Geometry: final body of the model. Coordinates: model frame, mm. A direction names the side the tool comes from. Give positions to 0.01 mm unless a question says otherwise; leave off trailing zeros. Write each loop counter-clockwise with the first axis right and the second up, starting at its lowest first coordinate (ties: lowest second). Pieces come first, ordered by that corner, then holes.
from build123d import *

# Parameters (mm, degrees)
SKETCH1_R           = 1.5
BOSS_EXTRUDE1_DEPTH = 3
SCALE1_SCALE        = 1.8


with BuildPart() as part:
    # Sketch1 → Boss-Extrude1 (new body)
    with BuildSketch(Plane(origin=(0, 0, 0), x_dir=(1, 0, 0), z_dir=(0, 1, 0))):
        with BuildLine():
            Line((0, -5), (23.998875872, -5))
            ThreePointArc((23.998875872, -5), (24.467345461, -4.883479623), (24.826642543, -4.561072489))
            Line((24.826642543, -4.561072489), (28.564941326, 0.954149161))
            ThreePointArc((28.564941326, 0.954149161), (28.766036178, 1.172359953), (29.022312673, 1.321950886))
            Line((29.022312673, 1.321950886), (40.929553216, 6.070049343))
            ThreePointArc((40.929553216, 6.070049343), (41.304486381, 6.141164834), (41.678758689, 6.066649533))
            Line((41.678758689, 6.066649533), (47.144586244, 3.829406729))
            Line((47.144586244, 3.829406729), (48.06174016, 3.086958957))
            Line((48.06174016, 3.086958957), (48.804187932, 4.004112872))
            Line((48.804187932, 4.004112872), (49.721341848, 3.2616651))
            Line((49.721341848, 3.2616651), (50.46378962, 4.178819016))
            Line((50.46378962, 4.178819016), (51.380943536, 3.436371244))
            Line((51.380943536, 3.436371244), (52.123391308, 4.35352516))
            Line((52.123391308, 4.35352516), (53.040545224, 3.611077387))
            Line((53.040545224, 3.611077387), (53.782992996, 4.528231303))
            Line((53.782992996, 4.528231303), (54.700146912, 3.785783531))
            Line((54.700146912, 3.785783531), (55.442594685, 4.702937447))
            Line((55.442594685, 4.702937447), (52.341745918, 12.244834503))
            ThreePointArc((52.341745918, 12.244834503), (52.137055639, 12.558350103), (51.831402108, 12.774604725))
            Line((51.831402108, 12.774604725), (46.024183924, 15.419882568))
            ThreePointArc((46.024183924, 15.419882568), (45.628323444, 15.509674561), (45.229386093, 15.434727162))
            Line((45.229386093, 15.434727162), (20.032711481, 5.075121772))
            ThreePointArc((20.032711481, 5.075121772), (19.846254378, 5.018960187), (19.652448068, 5))
            Line((19.652448068, 5), (0, 5))
            ThreePointArc((0, 5), (-5, 0), (0, -5))
        make_face()
        Circle(SKETCH1_R, mode=Mode.SUBTRACT)
        with Locations((22, 0)):
            Circle(SKETCH1_R, mode=Mode.SUBTRACT)
    extrude(amount=BOSS_EXTRUDE1_DEPTH)


with BuildPart() as part_1:
    # Scale1: scaled about (24.6084342, 1.5, -3.682524739)
    add(part.part.scale(SCALE1_SCALE).moved(Location((-19.68674736, -1.2, 2.946019791))))


solid = part_1.part
Q1. Section B-B on x = 10. Output: boundary loops of the cut face in (y, z), plus the area to 3 significant figures.
Filled sheet:
outline: (-1.2, -6.05) - (4.2, -6.05) - (4.2, 11.95) - (-1.2, 11.95) - close
area: 97.2 mm2
Q2. Section A-A on y = 2.95. Output: boundary loops of the cut face in (x, z).
Filled sheet:
outline: (-19.69, -6.05) - (15.69, -6.05) arc R1.8 cw to (16.37, -6.19) - (61.73, -24.84) arc R1.8 ccw to (63.16, -24.81) - (73.61, -20.05) arc R1.8 ccw to (74.53, -19.09) - (80.11, -5.52) - (78.77, -3.87) - (77.12, -5.2) - (75.79, -3.55) - (74.14, -4.89) - (72.8, -3.24) - (71.15, -4.58) - (69.81, -2.92) - (68.16, -4.26) - (66.82, -2.61) - (65.17, -3.95) - (55.34, -7.97) arc R1.8 cw to (53.99, -7.98) - (32.55, 0.57) arc R1.8 cw to (31.73, 1.23) - (25, 11.16) arc R1.8 ccw to (23.51, 11.95) - (-19.69, 11.95) arc R9 ccw to start; hole circle Ø5.4 at (-19.69, 2.95); hole circle Ø5.4 at (19.91, 2.95)
Q3. Ray query, line 1 along X through (y, z) = (2.6, 2.5); line 2 along Z through (x, y) = (-21.5, 1.8); line 3 along Z through (x, y) = (0.5, 2.35). Return the intervals inside material, ascending.
Filled sheet:
line 1: x = -28.68 to -22.35, -17.02 to 17.25, 22.58 to 30.87
line 2: z = -5.87 to 0.95, 4.95 to 11.76
line 3: z = -6.05 to 11.95
Q4. Access query for faces 1 (the cylindrical face through (-22.384, 1.462, 2.827)), 2 (the flat face through (-2, 1, -6.054)), 3 (the flat face through (43.12, 1.462, -3.647)). Directions: +Z, -Z, +X, -X, +Y, -Y. A direction counts if a zero-diameter tool reaches every point of the face in a straight line with its end or side. Return the directions, or none.
Filled sheet:
face 1: +Y, -Y
face 2: -Z, -X, +Y, -Y
face 3: +Z, +Y, -Y
Q5. Section C-C on z = -17. Output: boundary loops of the cut face in (x, y).
Filled sheet:
outline: (42.67, -1.2) - (75.39, -1.2) - (75.39, 4.2) - (42.67, 4.2) - close
Q6. Pin query (flat end, axial travel): P1, Ø1, axis at x = 31, y = 0.5, coming from the +Z side; P2, Ø7, axis at x = 19.91, z = 2.95, coming from the +Y side; P3, Ø2, axis at x = 36, y = 2, coming from the +Z side; P4, Ø3, axis at x = -19.69, z = 2.95, coming from the -Y side. Return the tip coordinate at first contact, or that it passes through.
Filled sheet:
P1: stops at z = 3.04
P2: stops at y = 4.2
P3: stops at z = -0.41
P4: passes through
